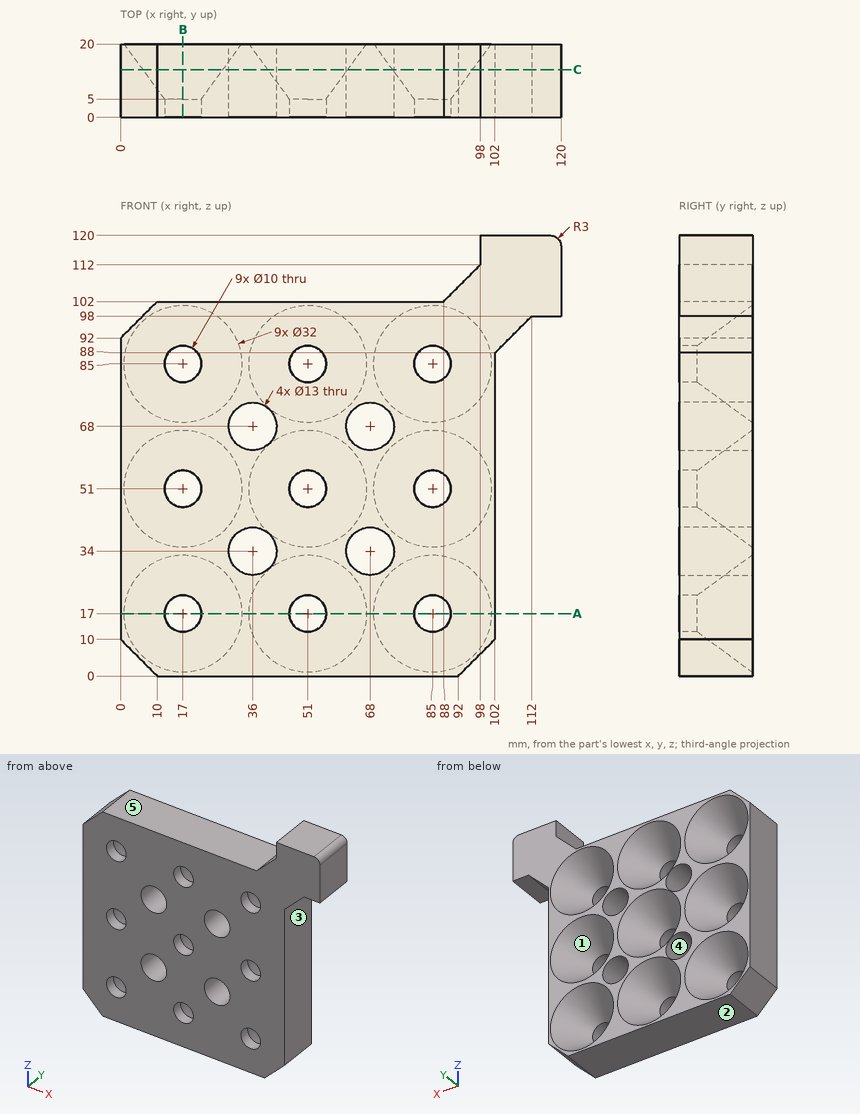
Answer from the drawing. Dimensions are ordinates in mm from the lowest x, y and z of the part. A direction names the side the tool comes from. Round coordinates to 2 decimals unless told otherwise and drop trailing zeros. Write each loop counter-clockwise with the first axis right and the second up, starting at its lowest first coordinate (ties: lowest second). Pieces come first, ordered by that corner, then holes. Notation, with made-up numbers: (-11, 87.25) - (26, 87.25) arc R17 ccw to (26, 113.25) - close; hole circle Ø7 at (35.25, -6.75). An arc over 180 degrees is marked (long way). Use a Markdown table: item, result.
(1) The mould has two halves that part along Z. Classify the marked faces 1, 2 and 3: released by +Z, released by -Z, zero draft, split by the parting line, or undercut.
Reported:
| item | result |
|---|---|
| face 1 | undercut |
| face 2 | released by -Z |
| face 3 | zero draft |
(2) Each of these flat-tipped pins is pushed along its axis until it touches: pin 1 Ø1 at (x, y) = (19.5, 2) entering from +Z; pin 2 Ø8 at (x, z) = (68, 34) entering from -Y; pin 3 Ø16 at (x, z) = (85, 51) entering from +Y; pin 4 Ø6.5 at (y, z) = (11.5, 115) entering from -X. Where does it stop, or does it pass through?
Reported:
| item | result |
|---|---|
| pin 1 | z = 102 |
| pin 2 | through |
| pin 3 | y = 9.09 |
| pin 4 | x = 97.75 |
(3) The part is cut by section A-A (z = 17). Write down the section's boundary in (x, y), then the cut area to 3 significant figures.
Reported:
| item | result |
|---|---|
| outline | (0, 0) - (12, 0) - (12, 5) - (1, 20) - (0, 20) - close; (22, 0) - (46, 0) - (46, 5) - (35, 20) - (33, 20) - (22, 5) - close; (56, 0) - (80, 0) - (80, 5) - (69, 20) - (67, 20) - (56, 5) - close; (90, 0) - (102, 0) - (102, 20) - (101, 20) - (90, 5) - close |
| area | 945 mm2 |
(4) The part is cut by section B-B (x = 17). Write down the section's boundary in (y, z).
Reported:
| item | result |
|---|---|
| outline | (0, 0) - (20, 0) - (20, 1) - (5, 12) - (0, 12) - close; (0, 22) - (5, 22) - (20, 33) - (20, 35) - (5, 46) - (0, 46) - close; (0, 56) - (5, 56) - (20, 67) - (20, 69) - (5, 80) - (0, 80) - close; (0, 90) - (5, 90) - (20, 101) - (20, 102) - (0, 102) - close |
(5) Straight lines are drawn through the part: line 1 along Z through (x, y) = (17, 1.4); line 2 along X through (y, z) = (14.25, 68). For each, find the intervals that lie inside material, in ascending order. Write a range as [from, to].
Reported:
| item | result |
|---|---|
| line 1 | [0, 12], [22, 46], [56, 80], [90, 102] |
| line 2 | [0, 29.5], [42.5, 61.5], [74.5, 102] |
(6) Which of the six approach directions +Z, -Z, +X, -X, +Y, -Y give full straight-line access (tool end or side, diameter ignored) to the marked faces 4 and 5?
Reported:
| item | result |
|---|---|
| face 4 | +Y, -Y |
| face 5 | +Z, -X, +Y, -Y |
(7) The part is cut by section C-C (y = 13). State how many separate pieces and enclosed holes the cut face has, then the cut area to 3 significant figures.
Reported:
| item | result |
|---|---|
| separate pieces | 1 |
| enclosed holes | 13 |
| area | 6,950 mm2 |
